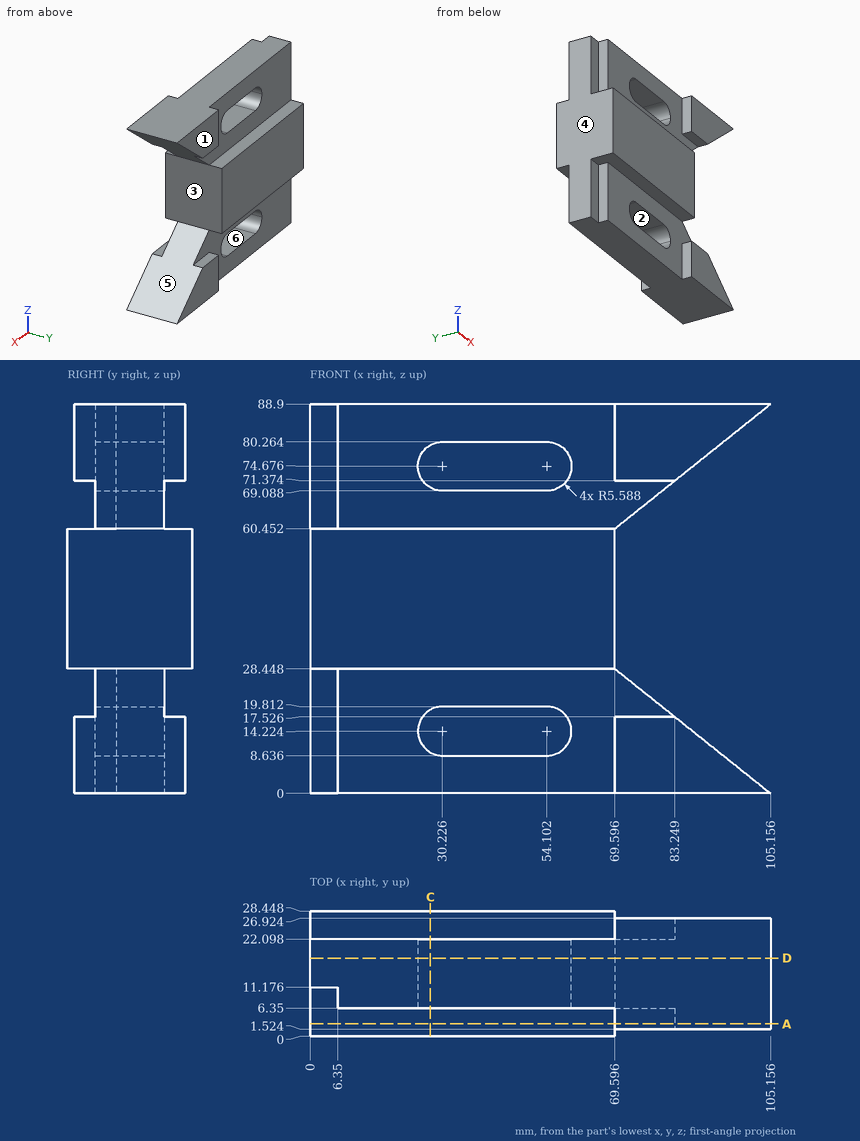
Geometry check sheet. Reference: drawing and pictorial views, mm from the part's lowest x, y, z. A direction names the side the tool comes from. Coordinates: 2 decimals unless noted, no trailing zeros. Loops run counter-clockwise (first coordinate to the right, second up) from the corner with the lowest first, then second, coordinate; pieces in that order, holes last. Notation, with made-up numbers: M -15,51.25 L 16,51.25 A21 ccw 16,81.25 Z; hole C 78,-33 d1. An arc over 180 degrees is marked long. One line per item, written item: value.
1. Set-up check for the marked faces 4, 5 and 6: record each of +Z, -Z, +X, -X, +Y, -Y from which the full face is reachable in a straight line by a thin tool's end or side.
Answers follow:
face 4: +Z, -Z, -X, +Y, -Y
face 5: +X, +Y, -Y
face 6: +Y, -Y
2. Section check D-D on y = 17.75. Record the cut outline in (x, z) (1 decimal).
Answers follow:
outline: M 0,0 L 105.2,0 L 69.6,28.4 L 69.6,60.5 L 105.2,88.9 L 0,88.9 Z; hole M 24.6,14.2 A5.6 ccw 30.2,8.6 L 54.1,8.6 A5.6 ccw 59.7,14.2 A5.6 ccw 54.1,19.8 L 30.2,19.8 A5.6 ccw Z; hole M 24.6,74.7 A5.6 ccw 30.2,69.1 L 54.1,69.1 A5.6 ccw 59.7,74.7 A5.6 ccw 54.1,80.3 L 30.2,80.3 A5.6 ccw Z
3. Material ranges on line 1 along Z through (x, y) = (76.5, 22.5) (1 decimal); line 2 along Y through (x, z) = (26, 61); line 3 along X through (y, z) = (6.5, 42) (1 decimal), recorded low to high. Write a range as from..to.
Answers follow:
line 1: 0..17.5, 71.4..88.9
line 2: 6.35..22.1
line 3: 0..69.6
4. Mould release check, pull along X, two halves, no side actions. Record for the marked faces 1, 2 and 3: pulls with the +X half, pulls with the -X half, needs draft (parallel to the pull), parting line crosses it, or undercut.
Answers follow:
face 1: needs draft
face 2: undercut
face 3: pulls with the +X half
5. Section check C-C on x = 27.5. Record the cut outline in (y, z).
Answers follow:
outline: M 0,28.45 L 6.35,28.45 L 6.35,19.1 L 22.1,19.1 L 22.1,28.45 L 28.45,28.45 L 28.45,60.45 L 22.1,60.45 L 22.1,69.8 L 6.35,69.8 L 6.35,60.45 L 0,60.45 Z; M 6.35,0 L 22.1,0 L 22.1,9.35 L 6.35,9.35 Z; M 6.35,79.55 L 22.1,79.55 L 22.1,88.9 L 6.35,88.9 Z
6. Gauge pin test, flat ends, axial feed: P1, Ø5, axis at y = 7, z = 54, coming from the +X side; P2, Ø3, axis at x = 2.5, z = 77.5, coming from the -Y side; P3, Ø1.4, axis at y = 8, z = 70, coming from the -X side. Record the tip position at first contact, or that the pin passes through.
Answers follow:
P1: x = 69.6
P2: y = 11.18
P3: x = 6.35
7. Section check A-A on y = 2.75. Record the cut outline in (x, z) (1 decimal), plus the area to 3 significant figures.
Answers follow:
outline: M 0,28.4 L 69.6,28.4 L 69.6,60.5 L 0,60.5 Z; M 69.6,0 L 105.2,0 L 83.2,17.5 L 69.6,17.5 Z; M 69.6,71.4 L 83.2,71.4 L 105.2,88.9 L 69.6,88.9 Z
area: 3,090 mm^2
